Print and shaded views of the part. All mm, measured from the part's lowest x, y and z. Give positions to 0.01 mm unless a question says otherwise; leave off trailing zeros. Loops run counter-clockwise (first coordinate to the right, second up) from the corner with the lowest first, then second, coordinate; pieces in that order, holes last. Notation, with made-up numbers: M 66,6.25 L 111,6.25 A30 ccw 111,30.25 Z; hole C 57,46.25 d8. An arc over 180 degrees is marked long. Answer in a Markdown table with one row per item.
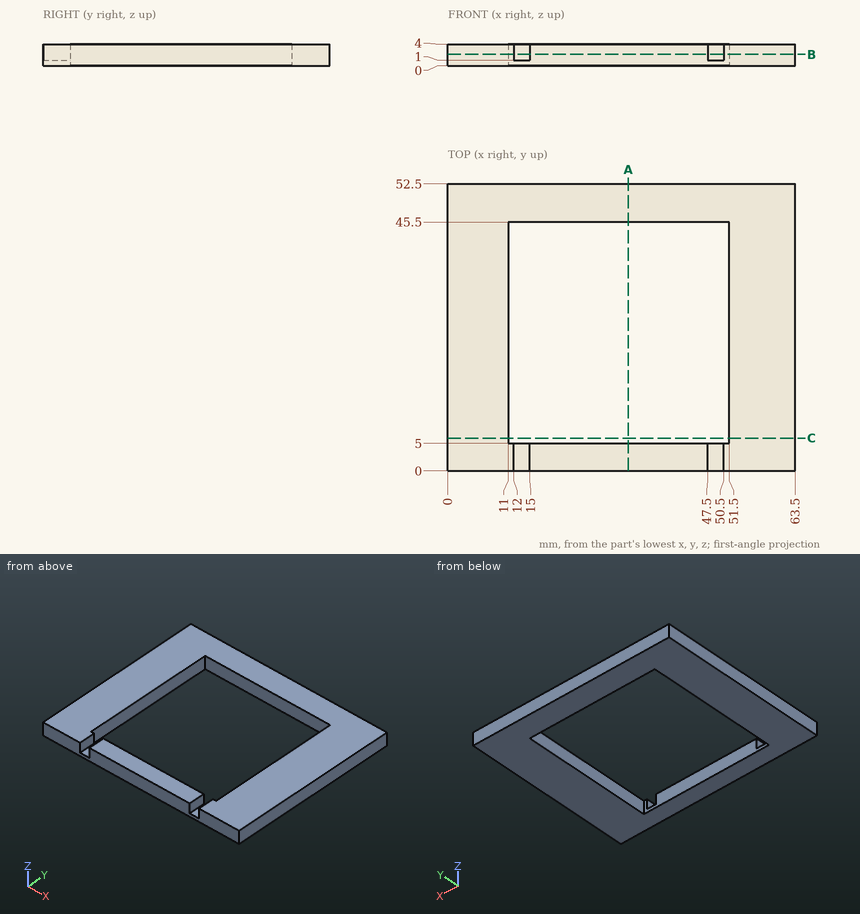
(1) Flat gauge pin, fed straight in: P1, Ø2.5, axis at x = 13.5, y = 3.5, coming from the +Z side. Where does the tip first touch, or does it go through?
Established:
| item | result |
|---|---|
| P1 | stops at z = 1 |
(2) Saw through at A-A, the plane x = 33. Give the cut face in (y, z), and give its area (3 significant figures).
Established:
| item | result |
|---|---|
| outline | M 0,0 L 5,0 L 5,4 L 0,4 Z; M 45.5,0 L 52.5,0 L 52.5,4 L 45.5,4 Z |
| area | 48.0 mm2 |
(3) Saw through at C-C, the plane y = 6. Give the cut face in (x, z).
Established:
| item | result |
|---|---|
| outline | M 0,0 L 11,0 L 11,4 L 0,4 Z; M 51.5,0 L 63.5,0 L 63.5,4 L 51.5,4 Z |
(4) Wall check: L1, parallel to X at y = 4, z = 3.05; L2, parallel to X at y = 40, z = 1.7; L3, parallel to Y at x = 41, z = 0.5. Give the ranges that are in metal, low to high.
Established:
| item | result |
|---|---|
| L1 | x = 0 to 12, 15 to 47.5, 50.5 to 63.5 |
| L2 | x = 0 to 11, 51.5 to 63.5 |
| L3 | y = 0 to 5, 45.5 to 52.5 |
(5) Saw through at B-B, the plane z = 2.1. Give the cut face in (x, y), and give its area (3 significant figures).
Established:
| item | result |
|---|---|
| outline | M 0,0 L 12,0 L 12,5 L 11,5 L 11,45.5 L 51.5,45.5 L 51.5,5 L 50.5,5 L 50.5,0 L 63.5,0 L 63.5,52.5 L 0,52.5 Z; M 15,0 L 47.5,0 L 47.5,5 L 15,5 Z |
| area | 1,660 mm2 |
